For this review, take the finished solid that the model builds, in its own axes (mm). Coordinates: 2 decimals unless noted, no trailing zeros.
```python
from build123d import *

# Parameters (mm, degrees)
F0_W     = 49.8404
F0_H     = 183.4444
F0_R     = 1.5
F1_DEPTH = 2
F2_R     = 4.75
F2_R_2   = 1.4732
F2_R_3   = 1.5
F3_DEPTH = 25
F4_W     = 2.45
F4_H     = 183.4444
F5_DEPTH = 0.4
F6_SIZE2 = 0.75
F6_SIZE  = 0.4330127019


with BuildPart() as f1:
    # F0 (on Top) → F1 (new body)
    with BuildSketch(Plane.XY):
        with Locations((21.9202, 88.7222)):
            Rectangle(F0_W, F0_H)
        Circle(F0_R, mode=Mode.SUBTRACT)
        with Locations((43.8404, 0)):
            Circle(F0_R, mode=Mode.SUBTRACT)
        with Locations((0, 177.4444)):
            Circle(F0_R, mode=Mode.SUBTRACT)
        with Locations((43.8404, 177.4444)):
            Circle(F0_R, mode=Mode.SUBTRACT)
    extrude(amount=-F1_DEPTH)

    # F2 (on face) → F3 (cut)
    with BuildSketch(Plane.XY):
        with Locations((10.5, 21.86895)):
            Circle(F2_R)
        with Locations((10.5, 5.15565)):
            Circle(F2_R)
        with Locations((27.264, 5.15565)):
            Circle(F2_R)
        with Locations((27.264, 21.86895)):
            Circle(F2_R)
        with Locations((10.5, 55.29555)):
            Circle(F2_R)
        with Locations((27.264, 55.29555)):
            Circle(F2_R)
        with Locations((10.5, 38.58225)):
            Circle(F2_R)
        with Locations((27.264, 38.58225)):
            Circle(F2_R)
        with Locations((10.5, 105.43545)):
            Circle(F2_R)
        with Locations((27.264, 105.43545)):
            Circle(F2_R)
        with Locations((27.264, 122.14875)):
            Circle(F2_R)
        with Locations((10.5, 122.14875)):
            Circle(F2_R)
        with Locations((27.264, 88.72215)):
            Circle(F2_R)
        with Locations((27.264, 72.00885)):
            Circle(F2_R)
        with Locations((10.5, 88.72215)):
            Circle(F2_R)
        with Locations((10.5, 72.00885)):
            Circle(F2_R)
        with Locations((27.264, 138.86205)):
            Circle(F2_R)
        with Locations((27.264, 172.28865)):
            Circle(F2_R)
        with Locations((27.264, 155.57535)):
            Circle(F2_R)
        with Locations((10.5, 138.86205)):
            Circle(F2_R)
        with Locations((10.5, 155.57535)):
            Circle(F2_R)
        with Locations((10.5, 172.28865)):
            Circle(F2_R)
        with Locations((43.8404, 0)):
            Circle(F2_R_2)
        with Locations((0, 177.4444)):
            Circle(F2_R_2)
        with Locations((33.5, 163.932)):
            Circle(F2_R_3)
        with Locations((15, 147.2187)):
            Circle(F2_R_3)
        with Locations((33.5, 130.5054)):
            Circle(F2_R_3)
        with Locations((15, 113.7921)):
            Circle(F2_R_3)
        with Locations((33.5, 97.0788)):
            Circle(F2_R_3)
        with Locations((15, 80.3655)):
            Circle(F2_R_3)
        with Locations((33.5, 63.6522)):
            Circle(F2_R_3)
        with Locations((15, 46.9389)):
            Circle(F2_R_3)
        with Locations((33.5, 30.2256)):
            Circle(F2_R_3)
        with Locations((15, 13.5123)):
            Circle(F2_R_3)
        Circle(F2_R_2)
        with Locations((43.8404, 177.4444)):
            Circle(F2_R_2)
    extrude(amount=-F3_DEPTH, mode=Mode.SUBTRACT)

    # F4 (on face) → F5 (cut)
    with BuildSketch(Plane.XY):
        with Locations((5.925, 88.7222)):
            Rectangle(F4_W, F4_H)
        with Locations((18.575, 88.7222)):
            Rectangle(F4_W, F4_H)
        with Locations((22.675, 88.7222)):
            Rectangle(F4_W, F4_H)
        with Locations((35.325, 88.7222)):
            Rectangle(F4_W, F4_H)
    extrude(amount=-F5_DEPTH, mode=Mode.SUBTRACT)

    # F6
    f6_edges = [f1.edges().sort_by_distance(p)[0] for p in [
        (46.8404, 88.7222, -2),
        (22.514, 5.15565, -2),
        (42.3404, 0, -2),
        (21.9202, -3, -2),
        (-1.5, 0, -2),
        (-3, 88.7222, -2),
        (5.75, 5.15565, -2),
        (13.5, 13.5123, -2),
        (22.514, 21.86895, -2),
        (32, 30.2256, -2),
        (5.75, 21.86895, -2),
        (5.75, 38.58225, -2),
        (22.514, 38.58225, -2),
        (22.514, 55.29555, -2),
        (32, 63.6522, -2),
        (22.514, 72.00885, -2),
        (5.75, 55.29555, -2),
        (13.5, 46.9389, -2),
        (5.75, 72.00885, -2),
        (13.5, 80.3655, -2),
        (22.514, 88.72215, -2),
        (32, 97.0788, -2),
        (5.75, 88.72215, -2),
        (22.514, 105.43545, -2),
        (5.75, 105.43545, -2),
        (13.5, 113.7921, -2),
        (22.514, 122.14875, -2),
        (32, 130.5054, -2),
        (5.75, 122.14875, -2),
        (22.514, 138.86205, -2),
        (5.75, 138.86205, -2),
        (22.514, 155.57535, -2),
        (32, 163.932, -2),
        (5.75, 155.57535, -2),
        (13.5, 147.2187, -2),
        (22.514, 172.28865, -2),
        (5.75, 172.28865, -2),
        (42.3404, 177.4444, -2),
        (21.9202, 180.4444, -2),
        (-1.5, 177.4444, -2),
    ]]
    f6_side = f1.faces().sort_by_distance((-1.099055, 88.7222, -2))[0]
    chamfer(f6_edges, length=F6_SIZE, length2=F6_SIZE2, reference=f6_side)


solid = f1.part
```
1) Consider section A-A (x = 10.5). Count the separate pieces of the cut face and the enclosed holes in it, then the cut area to 3 significant figures.
2) For L1, parallel to Y at x = 43.5, z = -1.1; L2, parallel to X at y = 105, z = -1.8; L3, parallel to X at y = 90, z = -1.2, list the stretches that pass through material, from the lowest coordinate up.
3) The part is to be moulded in two halves that separate along Y. For faces 1 (the face through (22, 90, -2)), 2 (the face through (32, 63.7, -0.8)), say which applies: pulls with the +Y half, pulls with the -Y half, needs draft (parallel to the pull), parting line crosses it, or undercut.
4) Clearance check with a flat-ended pin moving along its axis: P1, Ø3.5, axis at x = 15, y = 147.22, coming from the -Z side. State where the tip first meets the part, or that it passes through.
Results:
1. separate pieces: 12
1. enclosed holes: 0
1. area: 154 mm2
2. L1: y = -3 to -1.46, 1.46 to 175.98, 178.91 to 180.44
2. L2: x = -2.68 to 5.45, 15.55 to 22.22, 32.31 to 46.52
2. L3: x = -3 to 5.93, 15.07 to 22.69, 31.84 to 46.84
3. face 1: needs draft
3. face 2: undercut
4. P1: stops at z = -1.69
